```python
from build123d import *

# Parameters (mm, degrees)
F0_W     = 60
F0_H     = 60
F1_DEPTH = 25
F2_W     = 50
F2_H     = 50
F3_DEPTH = 20
F4_R     = 9.93
F4_R_2   = 7.43
F5_DEPTH = 43.3
F6_R     = 7.43
F7_DEPTH = 56.5
F8_R     = 5


with BuildPart() as f1:
    # F0 (on Top) → F1 (new body)
    with BuildSketch(Plane.XY):
        Rectangle(F0_W, F0_H)
    extrude(amount=F1_DEPTH)

    # F2 (on face) → F3 (cut)
    with BuildSketch(Plane.XY.offset(25)):
        Rectangle(F2_W, F2_H)
    extrude(amount=-F3_DEPTH, mode=Mode.SUBTRACT)

    # F4 (on face) → F5 (join)
    with BuildSketch(Plane.XY.offset(25)):
        Circle(F4_R)
        Circle(F4_R_2, mode=Mode.SUBTRACT)
    extrude(amount=-F5_DEPTH)

    # F6 (on face) → F7 (cut)
    with BuildSketch(Plane.XY.offset(25)):
        Circle(F6_R)
    extrude(amount=-F7_DEPTH, mode=Mode.SUBTRACT)

    # F8
    f8_edges = [f1.edges().sort_by_distance(p)[0] for p in [
        (-30, -30, 12.5),
        (30, -30, 12.5),
        (30, 30, 12.5),
        (-30, 30, 12.5),
    ]]
    fillet(f8_edges, radius=F8_R)


solid = f1.part
```
Here's how the part is built. I have some questions about the finished solid (model axes, mm). A direction names the side the tool comes from. Coordinates: 2 decimals unless noted, no trailing zeros. Order: outer loops, then holes, each group sorted by start corner. A loop starts at its lowest first (then second) coordinate and runs counter-clockwise, first axis right, second up.
1) Imagine slicing it at A-A on z = 12.5. List the corners of the cut face in (x, y) for me, and give its area (3 significant figures).
2) Imagine slicing it at B-B on x = 0. List the corners of the cut face in (y, z) for me.
3) I need wall thicknesses on line 1 (Y direction, x = 0, z = 8); line 2 (Y direction, x = 0, z = 2); line 3 (Y direction, x = 0, z = -6.5). Which ranges of each line are inside material? Lowest first, please.
4) We'd pull the mould along X, two halves only. Please class faces 4 (the face through (4, -7, 25)), 5 (the face through (0, 11, 5)), 6 (the face through (-28, -29, 13)), 7 (the face through (29, 28, 13)): +X half, -X half, draft (parallel to the pull), parting line (faces both ways), or undercut.
5) Imagine slicing it at D-D on z = 2. List the corners of the cut face in (x, y) for me, and give its area (3 significant figures).
6) Which directions (+Z, -Z, +X, -X, +Y, -Y) give clear straight access to the entire face, cutting with the end or side of a thin tool? Please do faces 1 (the face through (-2.153, -9.694, -9.022)), 2 (the face through (4, -7, -18.3)), 3 (the face through (-25, 0, 15)).
7) Will these pins go through, and if not, where does the flat tip stop? pin 1 (6 mm diameter, centred on x = -8.5, y = 21, fed in from +Z); pin 2 (2 mm diameter, centred on y = 0.5, z = -8, fed in from +X); pin 3 (8 mm diameter, centred on x = -10.5, z = -9, fed in from -Y).
Response values:
1. outline: (-30, -25) arc R5 ccw to (-25, -30) - (25, -30) arc R5 ccw to (30, -25) - (30, 25) arc R5 ccw to (25, 30) - (-25, 30) arc R5 ccw to (-30, 25) - close; circle Ø19.86 at (0, 0); hole (-25, -25) - (25, -25) - (25, 25) - (-25, 25) - close; hole circle Ø14.86 at (0, 0)
1. area: 1,210 mm2
2. outline: (-30, 0) - (-9.93, 0) - (-9.93, -18.3) - (-7.43, -18.3) - (-7.43, 25) - (-9.93, 25) - (-9.93, 5) - (-25, 5) - (-25, 25) - (-30, 25) - close; (7.43, -18.3) - (9.93, -18.3) - (9.93, 0) - (30, 0) - (30, 25) - (25, 25) - (25, 5) - (9.93, 5) - (9.93, 25) - (7.43, 25) - close
3. line 1: y = -30 to -25, -9.93 to -7.43, 7.43 to 9.93, 25 to 30
3. line 2: y = -30 to -7.43, 7.43 to 30
3. line 3: y = -9.93 to -7.43, 7.43 to 9.93
4. face 4: draft
4. face 5: undercut
4. face 6: -X half
4. face 7: +X half
5. outline: (-30, -25) arc R5 ccw to (-25, -30) - (25, -30) arc R5 ccw to (30, -25) - (30, 25) arc R5 ccw to (25, 30) - (-25, 30) arc R5 ccw to (-30, 25) - close; hole circle Ø14.86 at (0, 0)
5. area: 3,410 mm2
6. face 1: -Z
6. face 2: -Z, +X, -X, +Y, -Y
6. face 3: +Z
7. pin 1: stops at z = 5
7. pin 2: stops at x = 9.93
7. pin 3: stops at y = -7.51
